Read the model definition and answer for the solid it produces. Units are mm, in the model's axes. Face numbers are marked on the shaded views. A direction names the side the tool comes from. Coordinates: 2 decimals unless noted, no trailing zeros. Order: outer loops, then holes, each group sorted by start corner. A loop starts at its lowest first (then second) coordinate and runs counter-clockwise, first axis right, second up. Notation, with made-up numbers: M -26,46 L 26,46 A9 ccw 26,62 Z; hole C 88.5,-28 d8. An arc over 180 degrees is marked long. Use a Markdown table: item, result. Add a question column.
1) Find section B-B on z = 29.5. Write down the section's boundary in (x, y).
2) For the marked faces 4 and 5, determine the directions among +Z, -Z, +X, -X, +Y, -Y from which every point of the face is accessible in a straight line to the end or side of a thin tool.
3) Find section A-A on y = 8.25. Write down the section's boundary in (x, z).
4) Find the intervals of material crossed by probe 1 along X at (y, z) = (14.5, -12.5); probe 2 along Y at (x, z) = (5.5, 6); probe 3 along X at (y, z) = (6.5, -3), in increasing order. Write a range as [from, to].
5) Each of these flat-tipped pins is pushed along its axis until it touches: pin 1 Ø0.8 at (x, z) = (-34, 3) entering from +Y; pin 2 Ø3.5 at (x, z) = (-31, 17.5) entering from +Y; pin 3 Ø0.9 at (x, z) = (32, -7) entering from +Y; pin 4 Ø2 at (y, z) = (13.5, -24.5) entering from +X. Where does it stop, or does it pass through?
6) The mould has two halves that part along X. Classify the marked faces 1, 2 and 3: released by +X, released by -X, zero draft, split by the parting line, or undercut.
7) Find section C-C on x = 23. Write down the section's boundary in (y, z), plus the area to 3 significant figures.
Autodesk Inventor part; units mm, degrees
ref_plane "YZ Plane" through (0, 0, 0) normal (1, 0, 0) x (0, 1, 0)
ref_plane "XZ Plane" through (0, 0, 0) normal (0, 1, 0) x (-1, 0, 0)
ref_plane "XY Plane" through (0, 0, 0) normal (0, 0, 1) x (1, 0, 0)
sketch "Sketch1" plane through (0, 0, 0) normal (0, 1, 0) x (-1, 0, 0)
  line L0 (35, 40) -> (-35, 40)
  line L1 (-35, 40) -> (-35, -40)
  line L2 (-35, -40) -> (35, -40)
  line L3 (35, -40) -> (35, 40)
  line L4 (35, 40) -> (-35, -40) construction
  line L5 (-35, 40) -> (35, -40) construction
  point P0 (0, 0)
  dimension "d0" = 70
  dimension "d1" = 80
extrude "Extrusion1" add sketch "Sketch1" along normal blind 17.5
chamfer "Chamfer1" distance 5 angle 45 2 edges at (35, 0, 0) (-35, 0, 0)
shell "Shell1" thickness 5 removed faces 3 at (10, 11.6667, 40) at (11.6667, 17.5, 13.3333) at (-10, 11.6667, -40)
ref_plane "Work Plane1" through (0, 17.5, -40) normal (-1, 0, 0) x (0, 0, 1)
ref_plane "Work Plane2" through (-30, 0, 0) normal (0, 0, 1) x (1, 0, 0)
sketch "Sketch6" plane through (30, 17.5, 40) normal (1, 0, 0) x (0, 0, -1)
  line L0 (80, -12.5) -> (0, -12.5)
  line L1 (80, -12.5) -> (80, 0)
  line L2 (0, 0) -> (80, 0)
  line L3 (0, -12.5) -> (0, 0)
  line L4 (0, 0) -> (0, -10.4289)
  line L5 (0, -8) -> (80, -8)
  point P0 (40, -17.5)
  dimension "d31" = 8
extrude "Extrusion6" cut sketch "Sketch6" along normal blind 2.5 contours L5 L3 L2 L1
sketch "Sketch11" plane through (35, 17.5, 40) normal (1, 0, 0) x (0, 0, -1)
  line L0 (0, 9) -> (16.2241, 9)
  line L1 (0, 9) -> (0, 0)
  line L2 (0, 0) -> (27.1992, 0)
  line L3 (27.1992, 0) -> (30, -4)
  line L4 (30, -4) -> (50, -4)
  line L5 (50, -4) -> (52.8008, 0)
  line L6 (52.8008, 0) -> (80, 0)
  line L7 (80, 9) -> (80, 0)
  line L8 (63.7759, 9) -> (80, 9)
  line L9 (63.7759, 9) -> (60, 4.5)
  line L10 (20, 4.5) -> (60, 4.5)
  line L11 (20, 4.5) -> (16.2241, 9)
  line L12 (52.8008, 0) -> (27.1992, 0)
  line L13 (80, 0) -> (0, 0)
  point P0 (40, -17.5)
extrude "Extrusion11" cut sketch "Sketch11" against normal up to surface (2.5 mm away) contours L12 L5 L4 L3
fillet "Fillet3" radius 0.5 4 edges at (32.5, 17.5, -26.4004) (32.5, 17.5, 26.4004) (32.5, 13.5, -40) (32.5, 13.5, 40)
mirror "Mirror3" about plane through (0, 17.5, -40) normal (-1, 0, 0) of "Extrusion6", "Fillet3", "Extrusion11"
sketch "Sketch10" plane through (35, 17.5, 40) normal (1, 0, 0) x (0, 0, -1)
  circle A0 centre (15.4979, -4) radius 1.75
  circle A1 centre (64.5021, -4) radius 1.75
  point P0 (40, -17.5)
extrude "Extrusion10" cut sketch "Sketch10" against normal through all
sketch "Sketch12" plane through (-30, 0, 40) normal (0, 0, 1) x (1, 0, 0)
  line L0 (0, 9.5) -> (-3, 9.5)
  line L1 (-3, 17.5) -> (-3, 9.5)
  line L2 (-5, 17.5) -> (-3, 17.5)
  line L3 (-5, 5) -> (-5, 17.5)
  line L4 (0, 0) -> (-5, 5)
  line L5 (0, 0) -> (60, 0)
  line L6 (65, 5) -> (60, 0)
  line L7 (65, 5) -> (65, 17.5)
  line L8 (63, 17.5) -> (65, 17.5)
  line L9 (63, 9.5) -> (63, 17.5)
  line L10 (63, 9.5) -> (60, 9.5)
  line L11 (60, 9.5) -> (60, 7.0711)
  line L12 (60, 7.0711) -> (57.9289, 5)
  line L13 (57.9289, 5) -> (2.0711, 5)
  line L14 (2.0711, 5) -> (0, 7.0711)
  line L15 (0, 7.0711) -> (0, 9.5)
  line L16 (0, 0) -> (60, 0)
  line L17 (60, 0) -> (65, 0)
  line L18 (65, 0) -> (65, 5)
  point P0 (30, 0)
properties part number "A-02"
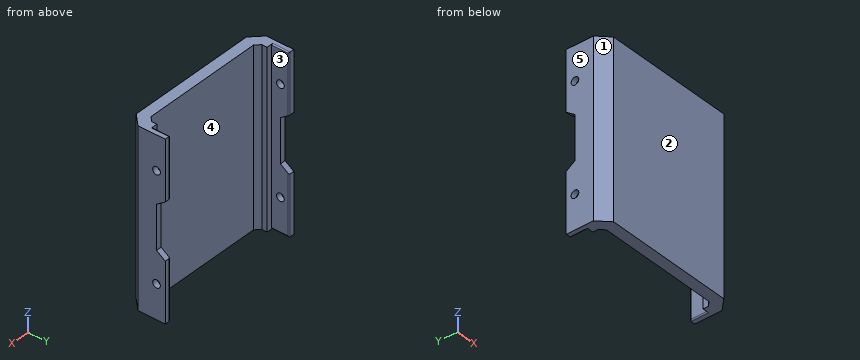
Check result:
| question | item | result |
|---|---|---|
| 1 | outline | M -35,5 L -30,0 L 30,0 L 35,5 L 35,17.5 L 33,17.5 A0.5 ccw 32.5,17 L 32.5,9.5 L 30,9.5 L 30,7.07 L 27.93,5 L -27.93,5 L -30,7.07 L -30,9.5 L -32.5,9.5 L -32.5,17 A0.5 ccw -33,17.5 L -35,17.5 Z |
| 2 | face 4 | +Z, -Z, +Y |
| 2 | face 5 | +Z, -Z, -X, +Y, -Y |
| 3 | outline | M -35,-40 L -30,-40 L -30,40 L -35,40 Z; M 30,-40 L 35,-40 L 35,40 L 30,40 Z |
| 4 | probe 1 | x = [-35, -32.5], [32.5, 35] |
| 4 | probe 2 | y = [0, 5] |
| 4 | probe 3 | x = [-35, -29.43], [29.43, 35] |
| 5 | pin 1 | stops at y = 13.5 |
| 5 | pin 2 | stops at y = 17.43 |
| 5 | pin 3 | stops at y = 9.5 |
| 5 | pin 4 | passes through |
| 6 | face 1 | released by -X |
| 6 | face 2 | zero draft |
| 6 | face 3 | undercut |
| 7 | outline | M 0,-40 L 5,-40 L 5,40 L 0,40 Z |
| 7 | area | 400 mm2 |
